```python
from build123d import *

# Parameters (mm, degrees)
SKETCH1_W                    = 97
SKETCH1_H                    = 75
BASE_FLANGE1_DEPTH           = 3.03784
EDGE_FLANGE1_STRIP_W         = 18.50136
EDGE_FLANGE1_STRIP_H         = 3.03784
EDGE_FLANGE1_STRIP_CUT_DEPTH = 75
EDGE_FLANGE1_DEPTH           = 75
EDGE_FLANGE2_DEPTH           = 50.78716
CUT_EXTRUDE3_DEPTH           = 134.298632329
M6_CLEARANCE_HOLE1_D         = 6.6


# Sheet-metal steps are written as plain solids
with BuildPart() as part:
    # Sketch1 → Base-Flange1 (new body)
    with BuildSketch(Plane.XY):
        with Locations((-48.5, 0)):
            Rectangle(SKETCH1_W, SKETCH1_H)
    extrude(amount=-BASE_FLANGE1_DEPTH)

    # Edge-Flange1 strip (across the edge) → Edge-Flange1 strip cut (cut)
    with BuildSketch(Plane(origin=(-97, -37.5, -3.03784), x_dir=(1, 0, 0), z_dir=(0, 1, 0))):
        with Locations((-3.03784, -1.51892)):
            Rectangle(EDGE_FLANGE1_STRIP_W, EDGE_FLANGE1_STRIP_H)
    extrude(amount=EDGE_FLANGE1_STRIP_CUT_DEPTH, mode=Mode.SUBTRACT)

    # Edge-Flange1 section (across the edge) → Edge-Flange1 (add)
    with BuildSketch(Plane(origin=(-97, -37.5, -3.03784), x_dir=(1, 0, 0), z_dir=(0, 1, 0))):
        with BuildLine():
            Line((0, 3.175), (0, 38.96216))
            Line((0, 38.96216), (3.03784, 38.96216))
            Line((3.03784, 38.96216), (3.03784, 3.175))
            ThreePointArc((3.03784, 3.175), (3.96777597, 0.92993597), (6.21284, 0))
            Line((6.21284, 0), (6.21284, -3.03784))
            ThreePointArc((6.21284, -3.03784), (1.819698706, -1.218141294), (0, 3.175))
        make_face()
    extrude(amount=EDGE_FLANGE1_DEPTH)

    # Edge-Flange2 section (across the edge) → Edge-Flange2 (add)
    with BuildSketch(Plane(origin=(-90.78716, 40.675, -3.03784), x_dir=(0, -1, 0), z_dir=(1, 0, 0))):
        with BuildLine():
            Line((-3.03784, 3.175), (-3.03784, 38.96216))
            Line((-3.03784, 38.96216), (0, 38.96216))
            Line((0, 38.96216), (0, 3.175))
            ThreePointArc((0, 3.175), (0.92993597, 0.92993597), (3.175, 0))
            Line((3.175, 0), (3.175, -3.03784))
            ThreePointArc((3.175, -3.03784), (-1.218141294, -1.218141294), (-3.03784, 3.175))
        make_face()
    extrude(amount=EDGE_FLANGE2_DEPTH)

    # Sketch13 → Cut-Extrude3 (cut, through all)
    with BuildSketch(Plane(origin=(0, 43.71284, 0), x_dir=(1, 0, 0), z_dir=(0, 1, 0))):
        with BuildLine():
            Line((-80.25, 37.25), (-80.25, 27.25))
            ThreePointArc((-80.25, 27.25), (-83, 24.5), (-85.75, 27.25))
            Line((-85.75, 27.25), (-85.75, 37.25))
            ThreePointArc((-85.75, 37.25), (-83, 40), (-80.25, 37.25))
        make_face()
        with BuildLine():
            Line((-55.25, 37.25), (-55.25, 27.25))
            ThreePointArc((-55.25, 27.25), (-58, 24.5), (-60.75, 27.25))
            Line((-60.75, 27.25), (-60.75, 37.25))
            ThreePointArc((-60.75, 37.25), (-58, 40), (-55.25, 37.25))
        make_face()
    extrude(amount=-CUT_EXTRUDE3_DEPTH, mode=Mode.SUBTRACT)

    # M6 Clearance Hole1 (through all)
    with Locations(Plane.XY):
        with Locations((-12, 23.71284), (-12, -26.28716), (-12, -1.28716)):
            Hole(M6_CLEARANCE_HOLE1_D / 2)


solid = part.part
```
Verification items for the finished model (mm, model axes). A direction names the side the tool comes from. Coordinates: 2 decimals unless noted, no trailing zeros. Loops run counter-clockwise (first coordinate to the right, second up) from the corner with the lowest first, then second, coordinate; pieces in that order, holes last. Notation, with made-up numbers: (9, 44) - (64, 44) arc R3 ccw to (64, 48) - close; hole circle Ø9 at (53, -12.75). An arc over 180 degrees is marked (long way). Answer as a JSON object with one key per item and string values.
(1) Scan lines: line 1 along Y through (x, z) = (-12, -1.5); line 2 along X through (y, z) = (-19, -15.5); line 3 along Z through (x, y) = (-49, -31.5). Record each from-to range of solid material in increasing order.
Response:
{"line 1": "y = -37.5 to -29.59, -22.99 to -4.59, 2.01 to 20.41, 27.01 to 37.5", "line 2": "x = -97 to -93.96", "line 3": "z = -3.04 to 0"}
(2) Cross-section at D-D, the plane z = -21. Record the boundary of the cut face in (x, y) (3 decimals), then the cut area to 3 significant figures.
Response:
{"outline": "(-97, -37.5) - (-93.962, -37.5) - (-93.962, 37.5) - (-97, 37.5) - close; (-90.787, 40.675) - (-40, 40.675) - (-40, 43.713) - (-90.787, 43.713) - close", "area": "382 mm²"}
(3) Mould release check, pull along X, two halves, no side actions. Record for faces 4 (the flat face through (-66, 43.713, -24)), 5 (the cylindrical face through (-82.9, 42.2, -24.5)), 6 (the flat face through (-90.787, 42, -21)): pulls with the +X half, pulls with the -X half, needs draft (parallel to the pull), parting line crosses it, or undercut.
Response:
{"face 4": "needs draft", "face 5": "undercut", "face 6": "pulls with the -X half"}
(4) Cross-section at A-A, the plane x = -12. Record the boundary of the cut face in (y, z), then the cut area to 3 significant figures.
Response:
{"outline": "(-37.5, -3.04) - (-29.59, -3.04) - (-29.59, 0) - (-37.5, 0) - close; (-22.99, -3.04) - (-4.59, -3.04) - (-4.59, 0) - (-22.99, 0) - close; (2.01, -3.04) - (20.41, -3.04) - (20.41, 0) - (2.01, 0) - close; (27.01, -3.04) - (37.5, -3.04) - (37.5, 0) - (27.01, 0) - close", "area": "168 mm²"}
(5) Cross-section at B-B, the plane z = -36. Record the boundary of the cut face in (x, y) (3 decimals), then the cut area to 3 significant figures.
Response:
{"outline": "(-97, -37.5) - (-93.962, -37.5) - (-93.962, 37.5) - (-97, 37.5) - close; (-90.787, 40.675) - (-85.75, 40.675) - (-85.75, 43.713) - (-90.787, 43.713) - close; (-80.25, 40.675) - (-60.75, 40.675) - (-60.75, 43.713) - (-80.25, 43.713) - close; (-55.25, 40.675) - (-40, 40.675) - (-40, 43.713) - (-55.25, 43.713) - close", "area": "349 mm²"}
(6) Go/stop test with flat-tipped pins: pin 1 Ø4 at (x, z) = (-68.5, -9) entering from -Y (3 decimals); pin 2 Ø1.9 at (y, z) = (42, -22.5) entering from -X; pin 3 Ø4 at (x, y) = (-69.5, 2) entering from -Z; pin 4 Ø4 at (x, y) = (-12, 23.71) entering from +Z. Record where each tip stops, or that it passes through.
Response:
{"pin 1": "stops at y = 40.675", "pin 2": "stops at x = -90.79", "pin 3": "stops at z = -3.04", "pin 4": "passes through"}
(7) Cross-section at C-C, the plane x = -83. Record the boundary of the cut face in (y, z) (3 decimals).
Response:
{"outline": "(-37.5, -3.038) - (37.5, -3.038) arc R3.175 cw to (40.675, -6.213) - (40.675, -24.5) - (43.713, -24.5) - (43.713, -6.213) arc R6.213 ccw to (37.5, 0) - (-37.5, 0) - close; (40.675, -42) - (43.713, -42) - (43.713, -40) - (40.675, -40) - close"}
(8) Access from +Z, -Z, +X, -X, +Y, -Y to the whole of each face (thin tool, end or side, straight path). Record for faces 1 (the flat face through (-20, 37.5, -2)), 2 (the flat face through (-60.75, 42, -32)), 3 (the flat face through (-95, 37.5, -21)).
Response:
{"face 1": "+Z, -Z, +X, +Y", "face 2": "+Y, -Y", "face 3": "+Z, -Z, -X, +Y"}
